Work out the finished part from the listing and answer in its coordinate system (mm). Coordinates: 2 decimals unless noted, no trailing zeros. Write each loop counter-clockwise with the first axis right and the second up, starting at its lowest first coordinate (ties: lowest second). Pieces come first, ordered by that corner, then holes. Notation, with made-up numbers: M 18.5,22 L 69.5,22 A38 cw 69.5,60 Z; hole C -33,17.25 d10. An arc over 180 degrees is marked long. Use CSV: the item, a comma, the result in double quotes.
from build123d import *

# Parameters (mm, degrees)
SKETCH1_R        = 3.25
MAIN_PLATE_DEPTH = 3


with BuildPart() as part:
    # Sketch1 → Main Plate (new body)
    with BuildSketch(Plane.XY):
        with BuildLine():
            Line((0, 75), (70, 75))
            ThreePointArc((70, 75), (77.071067812, 72.071067812), (80, 65))
            Line((80, 65), (80, -65))
            ThreePointArc((80, -65), (77.071067812, -72.071067812), (70, -75))
            Line((70, -75), (0, -75))
            ThreePointArc((0, -75), (-46.967889335, -58.472364168), (-73.235294118, -16.17379657))
            ThreePointArc((-73.235294118, -16.17379657), (-75.276849165, -11.977906289), (-79, -9.16515139))
            ThreePointArc((-79, -9.16515139), (-85, 0), (-79, 9.16515139))
            ThreePointArc((-79, 9.16515139), (-75.276849165, 11.977906289), (-73.235294118, 16.17379657))
            ThreePointArc((-73.235294118, 16.17379657), (-46.967889335, 58.472364168), (0, 75))
        make_face()
        with Locations((-75, 0)):
            Circle(SKETCH1_R, mode=Mode.SUBTRACT)
    extrude(amount=MAIN_PLATE_DEPTH)


solid = part.part
Item 1: Consider probe 1 along Y at (x, z) = (-75, 0.8); probe 2 along X at (y, z) = (19.5, 2); probe 3 along Y at (x, z) = (-55.5, 0.45). Determine where each line is inside the solid, lowest interval first.
Answer:
probe 1,"y = -12.33 to -3.25, 3.25 to 12.33"
probe 2,"x = -72.42 to 80"
probe 3,"y = -50.45 to 50.45"
Item 2: For a pull along Y with two mould halves and no side action, classify faces 1 (the face through (76.99, 72.15, 1.48)), 2 (the face through (17, 1, 0)), 3 (the face through (77.15, -71.99, 1.48)), 4 (the face through (-78.247, 0.143, 1.479)) as released by +Y, released by -Y, zero draft, split by the parting line, or undercut.
Answer:
face 1,"released by +Y"
face 2,"zero draft"
face 3,"released by -Y"
face 4,"undercut"
Item 3: Given pin 1 (1.5 mm diameter, centred on y = -43, z = 2, fed in from -X), flat-ended and moving along its own axis, determine where the tip first touches the part or whether it passes through.
Answer:
pin 1,"stops at x = -61.97"
Item 4: The part is cut by section C-C (x = -67.5). Write down the section's boundary in (y, z).
Answer:
outline,"M -32.69,0 L 32.69,0 L 32.69,3 L -32.69,3 Z"
Item 5: The part is cut by section A-A (y = 0). Write down the section's boundary in (x, z).
Answer:
outline,"M -85,0 L -78.25,0 L -78.25,3 L -85,3 Z; M -71.75,0 L 80,0 L 80,3 L -71.75,3 Z"
Item 6: The part is cut by section B-B (z = 1.4). Write down the section's boundary in (x, y), then the cut area to 3 significant figures.
Answer:
outline,"M -79,-9.17 A10 cw -73.24,-16.17 A75 ccw 0,-75 L 70,-75 A10 ccw 80,-65 L 80,65 A10 ccw 70,75 L 0,75 A75 ccw -73.24,16.17 A10 cw -79,9.17 A10 ccw Z; hole C -75,0 d6.5"
area,"20,900 mm2"
Item 7: The part is cut by section D-D (y = -24). Write down the section's boundary in (x, z).
Answer:
outline,"M -71.06,0 L 80,0 L 80,3 L -71.06,3 Z"
